from build123d import *

# Parameters (mm, degrees)
SKETCH1_W           = 73.025
SKETCH1_H           = 95.25
BOSS_EXTRUDE1_DEPTH = 3.175
SKETCH2_R           = 3.302
SKETCH2_W           = 50.8
SKETCH2_H           = 76.2
CUT_EXTRUDE1_DEPTH  = 3.81
SKETCH3_W           = 3.175
SKETCH3_H           = 3.175
BOSS_EXTRUDE2_DEPTH = 12.7


with BuildPart() as part:
    # Sketch1 → Boss-Extrude1 (new body)
    with BuildSketch(Plane.XY):
        with BuildLine():
            Line((-53.549611798, 36.126771133), (-53.549611798, -59.123228867))
            add(Edge.make_bspline(
                [(-53.549611798, 36.126771133), (-70.059671862, 7.530508267), (-74.046742033, -23.621157889), (-53.549611798, -59.123228867)],
                knots=[0, 0, 0, 0, 1, 1, 1, 1], degree=3))
        make_face()
        with Locations((-17.037111798, -11.498228867)):
            Rectangle(SKETCH1_W, SKETCH1_H)
        with Locations((55.987888202, -11.498228867)):
            Rectangle(SKETCH1_W, SKETCH1_H)
        with BuildLine():
            add(Edge.make_bspline(
                [(92.500388202, 36.126771133), (109.010448266, 7.530508267), (112.997518438, -23.621157889), (92.500388202, -59.123228867)],
                knots=[0, 0, 0, 0, 1, 1, 1, 1], degree=3))
            Line((92.500388202, -59.123228867), (92.500388202, 36.126771133))
        make_face()
    extrude(amount=BOSS_EXTRUDE1_DEPTH)

    # Sketch2 → Cut-Extrude1 (cut)
    with BuildSketch(Plane.XY.offset(3.175)):
        with Locations((-16.719611798, 0)):
            Circle(SKETCH2_R)
        with Locations((55.670388202, 0)):
            Circle(SKETCH2_R)
        with Locations((21.380388202, -9.593228867)):
            Rectangle(SKETCH2_W, SKETCH2_H)
        with BuildLine():
            Line((-49.077041311, 15.806771133), (-49.077041311, -34.993228867))
            add(Edge.make_bspline(
                [(-49.077041311, 15.806771133), (-57.589988192, 1.061914612), (-58.955244286, -17.883679426), (-49.077041311, -34.993228867)],
                knots=[0, 0, 0, 0, 1, 1, 1, 1], degree=3))
        make_face()
        with BuildLine():
            Line((88.027817715, 15.806771133), (88.027817715, -34.993228867))
            add(Edge.make_bspline(
                [(88.027817715, 15.806771133), (96.540764597, 1.061914612), (97.90602069, -17.883679426), (88.027817715, -34.993228867)],
                knots=[0, 0, 0, 0, 1, 1, 1, 1], degree=3))
        make_face()
    extrude(amount=-CUT_EXTRUDE1_DEPTH, mode=Mode.SUBTRACT)

    # Sketch3 → Boss-Extrude2 (add)
    with BuildSketch(Plane.XY.offset(3.175)):
        with Locations((-51.962111798, 34.539271133)):
            Rectangle(SKETCH3_W, SKETCH3_H)
        with Locations((-51.962111798, -57.535728867)):
            Rectangle(SKETCH3_W, SKETCH3_H)
        with Locations((90.912888202, -57.535728867)):
            Rectangle(SKETCH3_W, SKETCH3_H)
        with Locations((90.912888202, 34.539271133)):
            Rectangle(SKETCH3_W, SKETCH3_H)
    extrude(amount=BOSS_EXTRUDE2_DEPTH)


solid = part.part
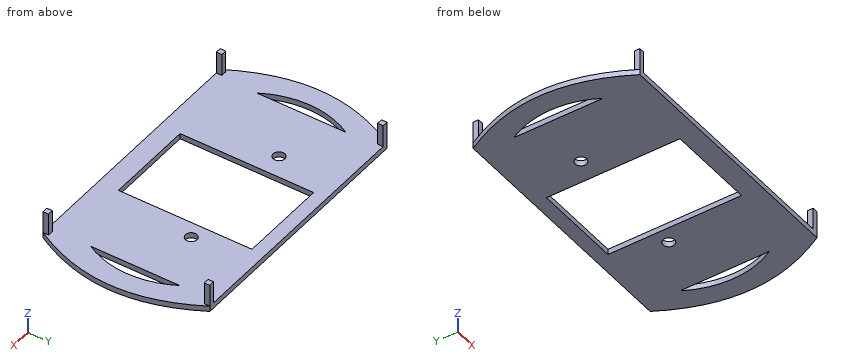
Input: part model. Units: mm. Frame: model coordinates. Coordinates: 2 decimals unless noted, no trailing zeros. Write each loop counter-clockwise with the first axis right and the second up, starting at its lowest first coordinate (ties: lowest second). Pieces come first, ordered by that corner, then holes. Notation, with made-up numbers: M -23.5,9.5 L 8.5,9.5 A29 cw 8.5,30.5 Z; hole C -6,-15 d1. An arc over 180 degrees is marked long. Answer as a JSON object with one key per item and string values. Group by question number.
(1) Section B-B on y = -12. Give the number of separate pieces and of enclosed holes in the cut face, plus the area to 3 significant figures.
(2) Section A-A on z = 14. Output: boundary loops of the cut face in (x, y).
(3) Ray query, line 1 along Y through (x, z) = (-53, 12); line 2 along Y through (x, z) = (5, 1); line 3 along X through (y, z) = (-16, 1.75). Return the intervals inside material, ascending. Write a range as [from, to].
(4) Contact query for flat-ended pins moving along their axis: P1, Ø1.6, axis at y = 35, z = 7, coming from the +X side; P2, Ø3.5, axis at y = -19.5, z = 2, coming from the +X side; P3, Ø1, axis at y = -58, z = 7.5, coming from the -X side; P4, Ø6, axis at x = 63, z = 7.5, coming from the -Y side. Output: stop coordinate, or through.
Result set:
{
 "1": {"separate pieces": "4", "enclosed holes": "0", "area": "347 mm2"},
 "2": {"outline": "M -53.55,-59.12 L -50.37,-59.12 L -50.37,-55.95 L -53.55,-55.95 Z; M -53.55,32.95 L -50.37,32.95 L -50.37,36.13 L -53.55,36.13 Z; M 89.33,-59.12 L 92.5,-59.12 L 92.5,-55.95 L 89.33,-55.95 Z; M 89.33,32.95 L 92.5,32.95 L 92.5,36.13 L 89.33,36.13 Z"},
 "3": {"line 1": "y = [-59.12, -55.95], [32.95, 36.13]", "line 2": "y = [-59.12, -47.69], [28.51, 36.13]", "line 3": "x = [-67.34, -55.58], [-49.08, -4.02], [46.78, 88.03], [94.53, 106.29]"},
 "4": {"P1": "stops at x = 92.5", "P2": "stops at x = 106.17", "P3": "stops at x = -53.55", "P4": "passes through"}
}
